Part model, mm, in its own coordinate system. A direction names the side the tool comes from. Coordinates: 2 decimals unless noted, no trailing zeros. Write each loop counter-clockwise with the first axis right and the second up, starting at its lowest first coordinate (ties: lowest second). Pieces come first, ordered by that corner, then holes. Notation, with made-up numbers: (71, 81.5) -> (86, 81.5) arc R11 ccw to (86, 86.5) -> close; hole circle Ø7 at (-6.75, 48.5). An arc over 180 degrees is marked (long way). Write item = value, one per line.
from build123d import *

# Parameters (mm, degrees)
SKETCH1_W          = 190
SKETCH1_H          = 125
SKETCH1_W_2        = 150
SKETCH1_H_2        = 85
EXTRUDE1_DEPTH     = 10
SKETCH2_W          = 16
SKETCH2_H          = 6
CUT_EXTRUDE1_DEPTH = 200
SKETCH3_R          = 1.6
SKETCH3_R_2        = 2.65
SKETCH3_R_3        = 2.5
CUT_EXTRUDE2_DEPTH = 20
SKETCH4_R          = 1.6
CUT_EXTRUDE3_DEPTH = 26
SKETCH5_R          = 2.75
CUT_EXTRUDE4_DEPTH = 10


with BuildPart() as part:
    # Sketch1 → Extrude1 (new body)
    with BuildSketch(Plane(origin=(0, 0, 0), x_dir=(1, 0, 0), z_dir=(0, 1, 0))):
        Rectangle(SKETCH1_W, SKETCH1_H)
        Rectangle(SKETCH1_W_2, SKETCH1_H_2, mode=Mode.SUBTRACT)
    extrude(amount=EXTRUDE1_DEPTH)

    # Sketch2 → Cut-Extrude1 (cut)
    with BuildSketch(Plane.ZY.offset(95)):
        with Locations((-52.5, 5)):
            Rectangle(SKETCH2_W, SKETCH2_H)
        with Locations((52.5, 5)):
            Rectangle(SKETCH2_W, SKETCH2_H)
    extrude(amount=-CUT_EXTRUDE1_DEPTH, mode=Mode.SUBTRACT)

    # Sketch3 → Cut-Extrude2 (cut)
    with BuildSketch(Plane(origin=(0, 10, 0), x_dir=(1, 0, 0), z_dir=(0, 1, 0))):
        with Locations((75, -52.5)):
            Circle(SKETCH3_R)
        with Locations((55, -52.5)):
            Circle(SKETCH3_R)
        with Locations((75, 52.5)):
            Circle(SKETCH3_R)
        with Locations((55, 52.5)):
            Circle(SKETCH3_R)
        with Locations((-55, 52.5)):
            Circle(SKETCH3_R)
        with Locations((-75, 52.5)):
            Circle(SKETCH3_R)
        with Locations((-75, -52.5)):
            Circle(SKETCH3_R)
        with Locations((-55, -52.5)):
            Circle(SKETCH3_R)
        with Locations((26.5, -52.5)):
            Circle(SKETCH3_R_2)
        with Locations((-26.5, -52.5)):
            Circle(SKETCH3_R_2)
        with Locations((15, 55.5)):
            Circle(SKETCH3_R_3)
        with Locations((-15, 55.5)):
            Circle(SKETCH3_R_3)
    extrude(amount=-CUT_EXTRUDE2_DEPTH, mode=Mode.SUBTRACT)

    # Sketch4 → Cut-Extrude3 (cut)
    with BuildSketch(Plane(origin=(0, 13, 0), x_dir=(1, 0, 0), z_dir=(0, 1, 0))):
        with Locations((90, 36)):
            Circle(SKETCH4_R)
        with Locations((80, 36)):
            Circle(SKETCH4_R)
        with Locations((90, -36)):
            Circle(SKETCH4_R)
        with Locations((80, -36)):
            Circle(SKETCH4_R)
        with Locations((-80, -36)):
            Circle(SKETCH4_R)
        with Locations((-90, -36)):
            Circle(SKETCH4_R)
        with Locations((-80, 36)):
            Circle(SKETCH4_R)
        with Locations((-90, 36)):
            Circle(SKETCH4_R)
    extrude(amount=-CUT_EXTRUDE3_DEPTH, mode=Mode.SUBTRACT)

    # Sketch5 → Cut-Extrude4 (cut)
    with BuildSketch(Plane(origin=(0, 10, 0), x_dir=(1, 0, 0), z_dir=(0, 1, 0))):
        with Locations((-87.5, -55)):
            Circle(SKETCH5_R)
        with Locations((-87.5, -30)):
            Circle(SKETCH5_R)
        with Locations((-87.5, 30)):
            Circle(SKETCH5_R)
        with Locations((-87.5, 55)):
            Circle(SKETCH5_R)
    extrude(amount=-CUT_EXTRUDE4_DEPTH, mode=Mode.SUBTRACT)


solid = part.part
Q1. Probe line 1 (Z direction, x = -15, y = 0.4); line 2 (Z direction, x = 72.5, y = 7.25); line 3 (X direction, y = 3, z = 30). List the from-to ranges inside material, lowest first. Write a range as from..to.
Model answer:
line_1 = -62.5..-58, -53..-42.5, 42.5..62.5
line_2 = -62.5..-60.5, -44.5..-42.5, 42.5..44.5, 60.5..62.5
line_3 = -95..-90.25, -84.75..-75, 75..95
Q2. Mould opens along X. For faces 1 (the face through (-1, 2, -53)), 2 (the face through (-75, 5, 1)), 3 (the face through (12.5, 9, -55.6)), 4 (the face through (95, 5, 1)) say: released by +X, released by -X, zero draft, split by the parting line, or undercut.
Model answer:
face_1 = zero draft
face_2 = undercut
face_3 = undercut
face_4 = released by +X
Q3. Which spindle directions (+Z, -Z, +X, -X, +Y, -Y) get a long thin tool onto all of the face, cutting with end or side? Do faces 5 (the face through (-87.858, 1.014, -57.727)), 6 (the face through (-1, 5, -60.5)). Say none if no direction does.
Model answer:
face_5 = +Y, -Y
face_6 = +X, -X
Q4. Saw through at A-A on y = 3.5. Count the separate pieces of the cut face and the enclosed holes in it, and give its area (3 significant figures).
Model answer:
separate_pieces = 3
enclosed_holes = 11
area = 4,810 mm²
Q5. Saw through at C-C on z = -30. Give the cut face in (x, y), and give its area (3 significant figures).
Model answer:
outline = (-95, 0) -> (-90.25, 0) -> (-90.25, 10) -> (-95, 10) -> close; (-84.75, 0) -> (-75, 0) -> (-75, 10) -> (-84.75, 10) -> close; (75, 0) -> (95, 0) -> (95, 10) -> (75, 10) -> close
area = 345 mm²
Q6. Saw through at B-B on x = 10.5. Give the cut face in (y, z), and give its area (3 significant figures).
Model answer:
outline = (0, -62.5) -> (10, -62.5) -> (10, -42.5) -> (0, -42.5) -> close; (0, 42.5) -> (10, 42.5) -> (10, 62.5) -> (0, 62.5) -> close; hole (2, -60.5) -> (8, -60.5) -> (8, -44.5) -> (2, -44.5) -> close; hole (2, 44.5) -> (8, 44.5) -> (8, 60.5) -> (2, 60.5) -> close
area = 208 mm²
Q7. Saw through at D-D on z = 46.5. Give the cut face in (x, y), and give its area (3 significant figures).
Model answer:
outline = (-95, 0) -> (95, 0) -> (95, 2) -> (-95, 2) -> close; (-95, 8) -> (95, 8) -> (95, 10) -> (-95, 10) -> close
area = 760 mm²
